Source: CAD feature listing. Evaluate the final solid. Frame: model axes, mm. A direction names the side the tool comes from. Give positions to 0.01 mm unless a question says otherwise; leave off trailing zeros. Order: outer loops, then holes, each group sorted by start corner. A loop starts at its lowest first (then second) coordinate and runs counter-clockwise, first axis right, second up.
from build123d import *

# Parameters (mm, degrees)
SKETCH_1_R      = 1
EXTRUDE_1_DEPTH = 1.5
SKETCH_3_R      = 3.5
SKETCH_3_R_2    = 2.490413186
EXTRUDE_2_DEPTH = 2


with BuildPart() as part:
    # 草图1 → 凸台-拉伸1 (new body)
    with BuildSketch(Plane(origin=(0, 0, 0), x_dir=(1, 0, 0), z_dir=(0, 1, 0))):
        with BuildLine():
            Line((-14.5, 2), (-1.319677425, 3.241674181))
            ThreePointArc((-1.319677425, 3.241674181), (3.5, 0), (-1.319677425, -3.241674181))
            Line((-1.319677425, -3.241674181), (-14.5, -2))
            ThreePointArc((-14.5, -2), (-16.5, 0), (-14.5, 2))
        make_face()
        with Locations(Location((-14.5, 0, 0), (0, 0, 270))):
            Circle(SKETCH_1_R, mode=Mode.SUBTRACT)
        with Locations(Location((0, 0, 0), (0, 0, 270))):
            Circle(SKETCH_1_R, mode=Mode.SUBTRACT)
    extrude(amount=EXTRUDE_1_DEPTH)

    # 草图3 → 凸台-拉伸2 (add)
    with BuildSketch(Plane(origin=(0, 1.5, 0), x_dir=(1, 0, 0), z_dir=(0, 1, 0))):
        with Locations(Location((0, 0, 0), (0, 0, 112.151115012))):
            Circle(SKETCH_3_R)
        with Locations(Location((0, 0, 0), (0, 0, 270))):
            Circle(SKETCH_3_R_2, mode=Mode.SUBTRACT)
    extrude(amount=EXTRUDE_2_DEPTH)


solid = part.part
1) Section query C-C on y = 1.75. Output: boundary loops of the cut face in (x, z), and give its area (3 significant figures).
Checks:
outline: circle Ø7 at (0, 0); hole circle Ø4.98 at (0, 0)
area: 19.0 mm2
2) Ray query, L1, parallel to X at y = 1.25, z = 0; L2, parallel to X at y = 2.6, z = 0; L3, parallel to Y at x = -7.5, z = 2.25. Return the intervals inside material, ascending.
Checks:
L1: x = -16.5 to -15.5, -13.5 to -1, 1 to 3.5
L2: x = -3.5 to -2.49, 2.49 to 3.5
L3: y = 0 to 1.5
3) First-contact query: pin 1 Ø1 at (x, y) = (-5, 0.5) entering from -Z. Flat tip, straight axial feed; report the tip coordinate or a pass-through.
Checks:
pin 1: stops at z = -2.94
4) Pull-direction query (Z, two-part tool) for faces 1 (the face through (-15.476, 0.74, -0.217)), 2 (the face through (-7.82, 0.74, 2.63)), 3 (the face through (2, 3.5, 2)); classes: +Z half, -Z half, draft (parallel to the pull), parting line (faces both ways), or undercut.
Checks:
face 1: undercut
face 2: +Z half
face 3: draft
5) Reachability of faces 4 (the face through (-8.002, 0.74, -2.612)), 5 (the face through (-1, 1.5, 1)) from +Z, -Z, +X, -X, +Y, -Y: full face, straight path, thin tool, end or side. Return the list, or none.
Checks:
face 4: -Z, -X, +Y, -Y
face 5: +Y
6) Section query B-B on z = 0. Output: boundary loops of the cut face in (x, y).
Checks:
outline: (-16.5, 0) - (-15.5, 0) - (-15.5, 1.5) - (-16.5, 1.5) - close; (-13.5, 0) - (-1, 0) - (-1, 1.5) - (-2.49, 1.5) - (-2.49, 3.5) - (-3.5, 3.5) - (-3.5, 1.5) - (-13.5, 1.5) - close; (1, 0) - (3.5, 0) - (3.5, 3.5) - (2.49, 3.5) - (2.49, 1.5) - (1, 1.5) - close
7) Section query A-A on x = 0. Output: boundary loops of the cut face in (y, z), and give its area (3 significant figures).
Checks:
outline: (0, -3.5) - (3.5, -3.5) - (3.5, -2.49) - (1.5, -2.49) - (1.5, -1) - (0, -1) - close; (0, 1) - (1.5, 1) - (1.5, 2.49) - (3.5, 2.49) - (3.5, 3.5) - (0, 3.5) - close
area: 11.5 mm2
8) Section query D-D on z = -2.25. Output: boundary loops of the cut face in (x, y), and give its area (3 significant figures).
Checks:
outline: (-11.85, 0) - (2.68, 0) - (2.68, 3.5) - (1.07, 3.5) - (1.07, 1.5) - (-1.07, 1.5) - (-1.07, 3.5) - (-2.68, 3.5) - (-2.68, 1.5) - (-11.85, 1.5) - close
area: 28.2 mm2
